Can you work these out from the model? Positions are in its coordinate system, mm. Face numbers are marked on the shaded views. A direction names the side the tool comes from. Give positions to 0.01 mm unless a question says otherwise; leave off trailing zeros. Loops run counter-clockwise (first coordinate to the right, second up) from the corner with the lowest first, then second, coordinate; pieces in that order, holes last.
from build123d import *

# Parameters (mm, degrees)
F0_R     = 3.175
F0_R_2   = 1.5875
F1_DEPTH = 2.54
F2_DEPTH = 25.4
F3_R     = 12.69999
F4_DEPTH = 31.75


# Not quite as in the source:
# - a fillet or chamfer is up to 0.001 mm smaller than in the source, because OpenCascade refuses the exact size


with BuildPart() as f1:
    # F0 (on Top) → F1 (new body)
    with BuildSketch(Plane.XY):
        Polygon((12.7, 167.64), (0, 167.64), (-12.7, 167.64), (-12.7, -12.7), (0, -12.7), (12.7, -12.7), align=None)
        Circle(F0_R, mode=Mode.SUBTRACT)
        with Locations((0, 154.94)):
            Circle(F0_R, mode=Mode.SUBTRACT)
        with Locations((0, 154.94)):
            Circle(F0_R)
        with Locations((0, 154.94)):
            Circle(F0_R_2, mode=Mode.SUBTRACT)
        with Locations((0, 154.94)):
            Circle(F0_R_2)
        Circle(F0_R)
        Circle(F0_R_2, mode=Mode.SUBTRACT)
        Circle(F0_R_2)
    extrude(amount=-F1_DEPTH)

    # F0 (on Top) → F2 (join)
    with BuildSketch(Plane.XY):
        with Locations((0, 154.94)):
            Circle(F0_R)
        with Locations((0, 154.94)):
            Circle(F0_R_2, mode=Mode.SUBTRACT)
        Circle(F0_R)
        Circle(F0_R_2, mode=Mode.SUBTRACT)
        with Locations((0, 154.94)):
            Circle(F0_R_2)
        Circle(F0_R_2)
    extrude(amount=F2_DEPTH)

    # F3 (radius 12.7 in the source; OpenCascade refuses exactly that, so slightly less here)
    f3_edges = [f1.edges().sort_by_distance(p)[0] for p in [
        (12.7, 167.64, -1.27),
        (-12.7, 167.64, -1.27),
        (-12.7, -12.7, -1.27),
        (12.7, -12.7, -1.27),
    ]]
    fillet(f3_edges, radius=F3_R)

    # F0 (on Top) → F4 (join)
    with BuildSketch(Plane.XY):
        Circle(F0_R_2)
        with Locations((0, 154.94)):
            Circle(F0_R_2)
    extrude(amount=F4_DEPTH)


solid = f1.part
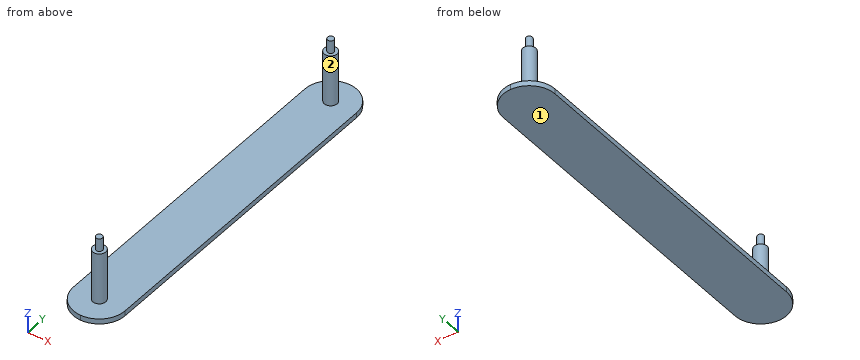
(1) Please list where these lines run through material, in increasing order: probe 1 along Z at (x, y) = (-5.5, 111); probe 2 along Y at (x, z) = (-1.75, 22.5); probe 3 along Y at (x, z) = (-1.25, 21).
Returned:
probe 1: z = -2.54 to 0
probe 2: y = -2.65 to 2.65, 152.29 to 157.59
probe 3: y = -2.92 to 2.92, 152.02 to 157.86
(2) Suppose I cut it at A-A on z = 20.5. List the corners of the cut face in (x, y) for me (3 decimals), plus the area to 3 significant figures.
Returned:
outline: circle Ø6.35 at (0, 0); circle Ø6.35 at (0, 154.94)
area: 63.3 mm2
(3) Suppose I cut it at B-B on y = 53. List the corners of the cut face in (x, z) for me.
Returned:
outline: (-12.7, -2.54) - (12.7, -2.54) - (12.7, 0) - (-12.7, 0) - close
(4) Suppose I cut it at C-C on z = 29. List the corners of the cut face in (x, y) for me (1 decimal).
Returned:
outline: circle Ø3.2 at (0, 0); circle Ø3.2 at (0, 154.9)
(5) Suppose I cut it at D-D on x = -9. List the corners of the cut face in (y, z) for me, plus the area to 3 significant figures.
Returned:
outline: (-8.96, -2.54) - (163.9, -2.54) - (163.9, 0) - (-8.96, 0) - close
area: 439 mm2
(6) Will these pins go through, and if not, where does the flat tip stop? P1, Ø6, axis at x = -0.5, z = 21.5, coming from the +Y side (3 decimals); P2, Ø1, axis at x = 7, y = 110, coming from the +Z side.
Returned:
P1: stops at y = 158.115
P2: stops at z = 0
(7) Which directions (+Z, -Z, +X, -X, +Y, -Y) give clear straight access to the entire face, cutting with the end or side of a thin tool? Please do the marked faces 1 and 2.
Returned:
face 1: -Z, +X, -X, +Y, -Y
face 2: +Z
